Here's the drawing with two shaded views (mm, measured from the low corner). I have some questions. A direction names the side the tool comes from. Coordinates: 2 decimals unless noted, no trailing zeros. Write each loop counter-clockwise with the first axis right and the second up, starting at its lowest first coordinate (ties: lowest second). Pieces come first, ordered by that corner, then holes.
Item 1: If I drill on probe 1 along Y at (x, z) = (64.5, 8); probe 2 along X at (y, z) = (62, 23.5); probe 3 along X at (y, z) = (38, 57), over which ranges is the centre line in solid material (lowest first)?
Item 2: I want a section at A-A on y = 27. Please give me the cut outline in (x, z).
Item 3: I want a section at D-D on y = 37. Please give me the cut outline in (x, z), then the cut area to 3 significant figures.
Item 4: Which directions (+Z, -Z, +X, -X, +Y, -Y) give clear straight access to the entire face, cutting with the end or side of a thin tool? Please do the marked faces 1, 2, 3, 4 and 5.
Item 5: For P1, Ø6, axis at x = 48, y = 60, coming from the -Z side; P2, Ø10.5, axis at y = 60, z = 47.5, coming from the +X side; P3, Ø7.5, axis at y = 44.5, z = 56.5, coming from the -X side, each with a flat end and sliding along its axis, tell me the tip position at first contact or that it passes through.
Item 6: I want a section at C-C on x = 49.5. Please give me the cut outline in (y, z).
Item 7: I want a section at B-B on z = 27. Please give me the cut outline in (x, y), then the cut area to 3 significant figures.
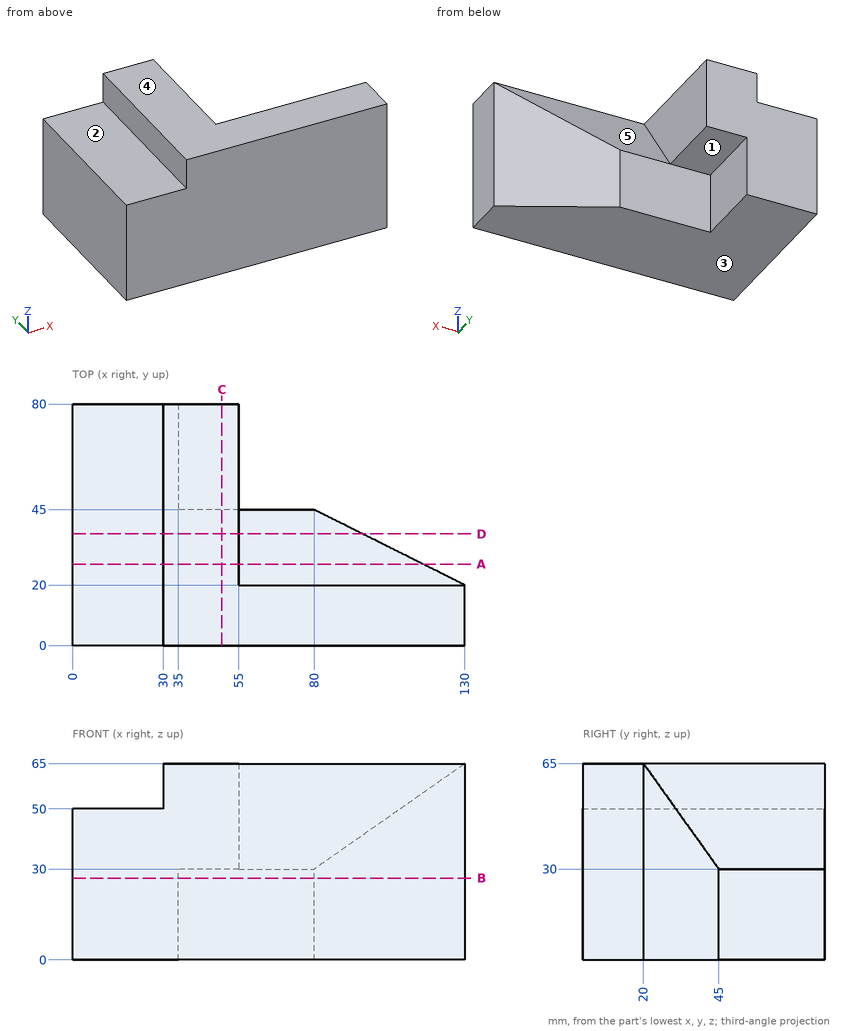
Response values:
1. probe 1: y = 0 to 45
1. probe 2: x = 0 to 35
1. probe 3: x = 30 to 55
2. outline: (0, 0) - (116, 0) - (116, 55.2) - (55, 55.2) - (55, 65) - (30, 65) - (30, 50) - (0, 50) - close
3. outline: (0, 0) - (96, 0) - (96, 41.2) - (55, 41.2) - (55, 65) - (30, 65) - (30, 50) - (0, 50) - close
3. area: 4,810 mm2
4. face 1: -Z, +X, +Y
4. face 2: +Z, -X, +Y, -Y
4. face 3: -Z, +X, -X, +Y, -Y
4. face 4: +Z, +X, -X, +Y, -Y
4. face 5: +Z, +X, +Y
5. P1: stops at z = 30
5. P2: stops at x = 55
5. P3: stops at x = 30
6. outline: (0, 0) - (45, 0) - (45, 30) - (80, 30) - (80, 65) - (0, 65) - close
7. outline: (0, 0) - (130, 0) - (130, 20) - (80, 45) - (35, 45) - (35, 80) - (0, 80) - close
7. area: 6,450 mm2
